```python
from build123d import *

# Parameters (mm, degrees)
F1_DEPTH = 4.5085
F2_R     = 3.175
F3_DEPTH = 4.7498
F4_R     = 1.778
F5_DEPTH = 25.4


with BuildPart() as f1:
    # F0 (on Front) → F1 (new body, symmetric)
    with BuildSketch(Plane.XZ):
        with BuildLine():
            Line((-7.9375, 11.1125), (-15.875, 11.1125))
            ThreePointArc((-15.875, 11.1125), (-23.732724, 7.857724), (-26.9875, 0))
            ThreePointArc((-26.9875, 0), (-23.732724, -7.857724), (-15.875, -11.1125))
            Line((-15.875, -11.1125), (0, -11.1125))
            Line((0, -11.1125), (15.875, -11.1125))
            ThreePointArc((15.875, -11.1125), (23.732724, -7.857724), (26.9875, 0))
            ThreePointArc((26.9875, 0), (23.732724, 7.857724), (15.875, 11.1125))
            Line((15.875, 11.1125), (7.9375, 11.1125))
            Line((7.9375, 11.1125), (7.9375, 4.7625))
            Line((7.9375, 4.7625), (0, 4.7625))
            Line((0, 4.7625), (-7.9375, 4.7625))
            Line((-7.9375, 4.7625), (-7.9375, 11.1125))
        make_face()
    extrude(amount=F1_DEPTH, both=True)

    # F2 (on face) → F3 (cut)
    with BuildSketch(Plane(origin=(0, 0, -11.1125), x_dir=(1, 0, 0), z_dir=(0, 0, -1))):
        with Locations((-4.445, 0)):
            Circle(F2_R)
        with Locations((4.445, 0)):
            Circle(F2_R)
    extrude(amount=-F3_DEPTH, mode=Mode.SUBTRACT)

    # F4 (on face) → F5 (cut)
    with BuildSketch(Plane(origin=(0, 0, -11.1125), x_dir=(1, 0, 0), z_dir=(0, 0, -1))):
        with Locations((-4.445, 0)):
            Circle(F4_R)
        with Locations((4.445, 0)):
            Circle(F4_R)
    extrude(amount=-F5_DEPTH, mode=Mode.SUBTRACT)


solid = f1.part
```
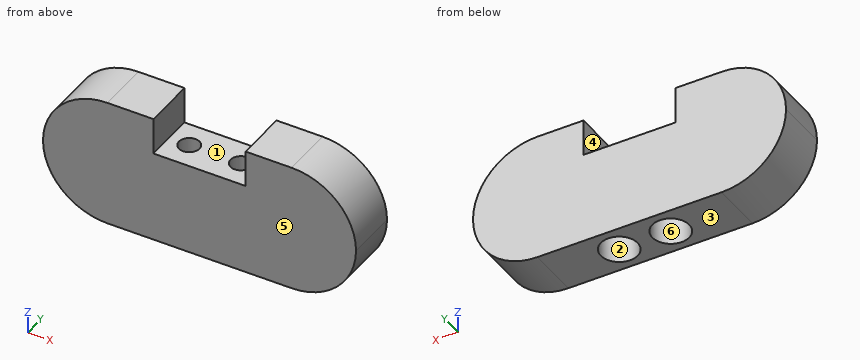
Here's how the part is built. I have some questions about the finished solid (model axes, mm). Face numbers are marked on the shaded views. A direction names the side the tool comes from. Coordinates: 2 decimals unless noted, no trailing zeros. Order: outer loops, then holes, each group sorted by start corner. A loop starts at its lowest first (then second) coordinate and runs counter-clockwise, first axis right, second up. Notation, with made-up numbers: (-14, 25) - (14, 25) arc R22 ccw to (14, 47) - close; hole circle Ø3 at (-28.75, 64.5). An arc over 180 degrees is marked (long way). One line per question, with ' | ' between items. Start each with the question number.
1. If we section it at A-A (y = 0): Write out the boundary of the cut face in (x, z) (1 decimal).
2. Which directions (+Z, -Z, +X, -X, +Y, -Y) give clear straight access to the entire face, cutting with the end or side of a thin tool? Please do the marked faces 1, 2 and 3.
3. If we section it at D-D (z = 3.75): Write out the boundary of the cut face in (x, y) (1 decimal).
4. If we section it at B-B (z = 9): Write out the boundary of the cut face in (x, y).
5. Please list where these lines run through material, in increasing order: line 1 along X through (y, z) = (0, -0.5); line 2 along X through (y, z) = (0, -9); line 3 along Z through (x, y) = (7, -2.25). Write a range as [from, to].
6. If we section it at C-C (x = 5.5): Write out the boundary of the cut face in (y, z).
7. I'm going to push flat-ended pins straight in: pin 1 Ø1.9 at (y, z) = (0.5, 8) entering from -X; pin 2 Ø4 at (x, y) = (-4.445, 0) entering from +Z; pin 3 Ø2 at (y, z) = (1.5, -3) entering from +X. Where does each tip first touch, or does it pass through?
8. If we mould it in two halves opening along X, with no side actions, what happens to the marked faces 4, 5 and 6? For each: released by +X, released by -X, zero draft, split by the parting line, or undercut.
Model answer:
1) outline: (-15.9, -11.1) - (-7.6, -11.1) - (-7.6, -6.4) - (-6.2, -6.4) - (-6.2, 4.8) - (-7.9, 4.8) - (-7.9, 11.1) - (-15.9, 11.1) arc R11.1 ccw to start; (-2.7, -6.4) - (-1.3, -6.4) - (-1.3, -11.1) - (1.3, -11.1) - (1.3, -6.4) - (2.7, -6.4) - (2.7, 4.8) - (-2.7, 4.8) - close; (6.2, -6.4) - (7.6, -6.4) - (7.6, -11.1) - (15.9, -11.1) arc R11.1 ccw to (15.9, 11.1) - (7.9, 11.1) - (7.9, 4.8) - (6.2, 4.8) - close
2) face 1: +Z, +Y, -Y | face 2: -Z | face 3: -Z, +X, -X, +Y, -Y
3) outline: (-26.3, -4.5) - (26.3, -4.5) - (26.3, 4.5) - (-26.3, 4.5) - close; hole circle Ø3.6 at (-4.4, 0); hole circle Ø3.6 at (4.4, 0)
4) outline: (-22.39, -4.51) - (-7.94, -4.51) - (-7.94, 4.51) - (-22.39, 4.51) - close; (7.94, -4.51) - (22.39, -4.51) - (22.39, 4.51) - (7.94, 4.51) - close
5) line 1: x = [-26.98, -6.22], [-2.67, 2.67], [6.22, 26.98] | line 2: x = [-22.39, -7.62], [-1.27, 1.27], [7.62, 22.39] | line 3: z = [-11.11, 4.76]
6) outline: (-4.51, -11.11) - (-2.99, -11.11) - (-2.99, -6.36) - (-1.43, -6.36) - (-1.43, 4.76) - (-4.51, 4.76) - close; (1.43, -6.36) - (2.99, -6.36) - (2.99, -11.11) - (4.51, -11.11) - (4.51, 4.76) - (1.43, 4.76) - close
7) pin 1: stops at x = -24.46 | pin 2: stops at z = 4.76 | pin 3: stops at x = 26.81
8) face 4: undercut | face 5: zero draft | face 6: undercut
